Design review of the part built by this model. Coordinates are the model's own, in mm. Face numbers are marked on the shaded views. Give positions to 0.01 mm unless a question says otherwise; leave off trailing zeros. Loops run counter-clockwise (first coordinate to the right, second up) from the corner with the lowest first, then second, coordinate; pieces in that order, holes last. Notation, with made-up numbers: (48, 88) - (52, 88) arc R33 cw to (52, 126) - close; hole circle Ø7 at (42.25, -1.5). An arc over 180 degrees is marked (long way). Write each question's results on one line, items separated by ' | '.
from build123d import *

# Parameters (mm, degrees)
SKETCH_R        = 30
PAD_DEPTH       = 30
SKETCH001_W     = 80
SKETCH001_H     = 80
PAD001_DEPTH    = 3
SKETCH002_R     = 28
POCKET_DEPTH    = 53
SKETCH003_R     = 3
POCKET001_DEPTH = 3
FILLET_R        = 6


with BuildPart() as part:
    # Sketch → Pad (new body)
    with BuildSketch(Plane.XY):
        Circle(SKETCH_R)
    extrude(amount=PAD_DEPTH)

    # Sketch001 → Pad001 (join)
    with BuildSketch(Plane.XY):
        Rectangle(SKETCH001_W, SKETCH001_H)
    extrude(amount=PAD001_DEPTH)

    # Sketch002 (on Face9 of Pad001) → Pocket (cut)
    with BuildSketch(Plane.XY.offset(30)):
        Circle(SKETCH002_R)
    extrude(amount=-POCKET_DEPTH, mode=Mode.SUBTRACT)

    # Sketch003 (on Face2 of Pocket) → Pocket001 (cut)
    with BuildSketch(Plane(origin=(0, 0, 0), x_dir=(1, 0, 0), z_dir=(0, 0, -1))):
        with Locations((-30, 30)):
            Circle(SKETCH003_R)
        with Locations((30, 30)):
            Circle(SKETCH003_R)
        with Locations((30, -30)):
            Circle(SKETCH003_R)
        with Locations((-30, -30)):
            Circle(SKETCH003_R)
    extrude(amount=-POCKET001_DEPTH, mode=Mode.SUBTRACT)

    # Fillet
    fillet_edges = [part.edges().sort_by_distance(p)[0] for p in [
        (-40, -40, 1.5),
        (40, -40, 1.5),
        (40, 40, 1.5),
        (-40, 40, 1.5),
    ]]
    fillet(fillet_edges, radius=FILLET_R)


solid = part.part
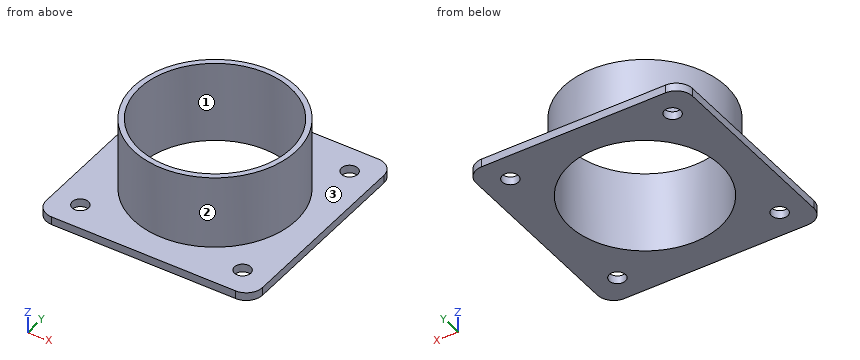
(1) Wall thickness on line 1 along X through (y, z) = (30, 1.9); line 2 along Y through (x, z) = (0, 17): over which ranges is each line inside the solid? List them lowest first. Write a range as from..to.
Answers below:
line 1: -40..-33, -27..27, 33..40 | line 2: -30..-28, 28..30
(2) Draft analysis for pull direction X (two halves, no side actions). For the marked faces 1, 2 and 3, state which applies: pulls with the +X half, pulls with the -X half, needs draft (parallel to the pull), parting line crosses it, or undercut.
Answers below:
face 1: undercut | face 2: parting line crosses it | face 3: needs draft
(3) Take a section at C-C on z = 26.75. Give the boundary of the cut face in (x, y).
Answers below:
outline: circle Ø60 at (0, 0); hole circle Ø56 at (0, 0)
(4) Take a section at B-B on x = 24.5. Give the boundary of the cut face in (y, z), plus the area to 3 significant figures.
Answers below:
outline: (-40, 0) - (-13.56, 0) - (-13.56, 30) - (-17.31, 30) - (-17.31, 3) - (-40, 3) - close; (13.56, 0) - (40, 0) - (40, 3) - (17.31, 3) - (17.31, 30) - (13.56, 30) - close | area: 362 mm2
(5) Take a section at A-A on y = 0. Give the boundary of the cut face in (x, z), plus the area to 3 significant figures.
Answers below:
outline: (-40, 0) - (-28, 0) - (-28, 30) - (-30, 30) - (-30, 3) - (-40, 3) - close; (28, 0) - (40, 0) - (40, 3) - (30, 3) - (30, 30) - (28, 30) - close | area: 180 mm2
(6) Insertion check: P1, Ø3, axis at x = 23.5, z = 5, coming from the +Y side; P2, Ø12, axis at y = 6, z = 24, coming from the -X side; P3, Ø3, axis at x = 25, z = 22.5, coming from the +Y side. Each pin has a flat end and moves straight along its axis. Give the tip position at first contact, or say it passes through.
Answers below:
P1: y = 20.4 | P2: x = -30 | P3: y = 18.65
